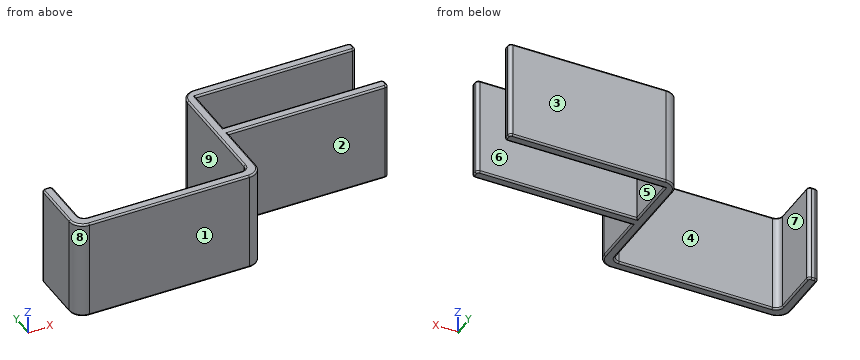
from build123d import *

# Parameters (mm, degrees)
PAD_DEPTH = 30
FILLET_R  = 0.5


with BuildPart() as part:
    # Sketch → Pad (new body)
    with BuildSketch(Plane(origin=(0, 0, 0), x_dir=(-1, 0, 0), z_dir=(0, 0, 1))):
        with BuildLine():
            ThreePointArc((1, 23), (-1.828427, 21.828427), (-3, 19))
            Line((-3, 3), (-3, 19))
            Line((-3, 3), (-49.999999, 3))
            ThreePointArc((-49.999999, 3), (-50.707106, 2.707107), (-50.999999, 2))
            Line((-50.999999, 1), (-50.999999, 2))
            ThreePointArc((-50.999999, 1), (-50.707106, 0.292893), (-49.999999, 0))
            Line((-3, 0), (-49.999999, 0))
            Line((-3, -16), (-3, 0))
            Line((-3, -16), (-49.999999, -16))
            ThreePointArc((-49.999999, -16), (-50.707106, -16.292893), (-50.999999, -17))
            Line((-50.999999, -18), (-50.999999, -17))
            ThreePointArc((-50.999999, -18), (-50.707106, -18.707107), (-49.999999, -19))
            Line((-4, -19), (-49.999999, -19))
            ThreePointArc((-4, -19), (-1.171573, -17.828427), (0, -15))
            Line((0, -15), (0, 18))
            ThreePointArc((2, 20), (0.585786, 19.414214), (0, 18))
            Line((2, 20), (48, 20))
            ThreePointArc((50, 18), (49.414214, 19.414214), (48, 20))
            Line((50, 18), (50, 4))
            ThreePointArc((50, 4), (50.292893, 3.292893), (51, 3))
            Line((52, 3), (51, 3))
            ThreePointArc((52, 3), (52.707107, 3.292893), (53, 4))
            Line((53, 19), (53, 4))
            ThreePointArc((53, 19), (51.828427, 21.828427), (49, 23))
            Line((1, 23), (49, 23))
        make_face()
    extrude(amount=PAD_DEPTH)

    # Fillet
    fillet_edges = [part.edges().sort_by_distance(p)[0] for p in [
        (-51.828427, -21.828427, 0),
        (-25, -23, 0),
        (1.828427, -21.828427, 0),
        (3, -11, 0),
        (26.5, -3, 0),
        (50.707106, -2.707107, 0),
        (50.999999, -1.5, 0),
        (50.707106, -0.292893, 0),
        (26.5, 0, 0),
        (3, 8, 0),
        (26.5, 16, 0),
        (50.707106, 16.292893, 0),
        (50.999999, 17.5, 0),
        (50.707106, 18.707107, 0),
        (27, 19, 0),
        (1.171573, 17.828427, 0),
        (0, -1.5, 0),
        (-0.585786, -19.414214, 0),
        (-25, -20, 0),
        (-49.414214, -19.414214, 0),
        (-50, -11, 0),
        (-50.292893, -3.292893, 0),
        (-51.5, -3, 0),
        (-52.707107, -3.292893, 0),
        (-53, -11.5, 0),
        (-51.828427, -21.828427, 30),
        (-25, -23, 30),
        (1.828427, -21.828427, 30),
        (3, -11, 30),
        (26.5, -3, 30),
        (50.707106, -2.707107, 30),
        (50.999999, -1.5, 30),
        (50.707106, -0.292893, 30),
        (26.5, 0, 30),
        (3, 8, 30),
        (26.5, 16, 30),
        (50.707106, 16.292893, 30),
        (50.999999, 17.5, 30),
        (50.707106, 18.707107, 30),
        (27, 19, 30),
        (1.171573, 17.828427, 30),
        (0, -1.5, 30),
        (-0.585786, -19.414214, 30),
        (-25, -20, 30),
        (-49.414214, -19.414214, 30),
        (-50, -11, 30),
        (-50.292893, -3.292893, 30),
        (-51.5, -3, 30),
        (-52.707107, -3.292893, 30),
        (-53, -11.5, 30),
    ]]
    fillet(fillet_edges, radius=FILLET_R)


solid = part.part
Check sheet for the modelled part. Datum: model origin and axes. Units: mm. Face numbers are marked on the shaded views. A direction names the side the tool comes from. Give positions to 0.01 mm unless a question says otherwise; leave off trailing zeros. Loops run counter-clockwise (first coordinate to the right, second up) from the corner with the lowest first, then second, coordinate; pieces in that order, holes last. Notation, with made-up numbers: M -8,4 L 38,4 A31 ccw 38,28 Z; hole C -2.75,40 d9. An arc over 180 degrees is marked long. Answer as a JSON object with one key per item and string values. Group by question number.
Q1. Cross-section at D-D on x = -26. Record the cut outline in (y, z).
Q2. Cross-section at A-A on y = -9.5. Record the cut outline in (x, z), then the cut area to 3 significant figures.
Q3. Cross-section at C-C on z = 22.5. Record the cut outline in (x, y), then the cut area to 3 significant figures.
Q4. Cross-section at B-B on x = 29. Record the cut outline in (y, z), then the cut area to 3 significant figures.
Q5. Release check for a two-part mould opening along X. For the marked faces 6, 7, 8 and 9 record: released by +X, released by -X, zero draft, split by the parting line, or undercut.
Q6. Access from +Z, -Z, +X, -X, +Y, -Y to the whole of each face (thin tool, end or side, straight path). Record for the marked faces 1, 2, 3, 4 and 5.
Q7. Material ranges on line 1 along Y through (x, z) = (33, 1.5); line 2 along X through (y, z) = (-10.5, 17.5); line 3 along X through (y, z) = (7.5, 20.25), recorded low to high. Write a range as [from, to].
Q8. Go/stop test with flat-tipped pins: P1, Ø14.5, axis at x = 24.5, z = 15.5, coming from the -Y side; P2, Ø6, axis at y = 12.5, z = 7.5, coming from the +X side; P3, Ø1.1, axis at x = -51.5, z = 9.5, coming from the +Y side. Record where each tip stops, or that it passes through.
Evaluation:
{
 "1": {"outline": "M -23,0.5 A0.5 ccw -22.5,0 L -20.5,0 A0.5 ccw -20,0.5 L -20,29.5 A0.5 ccw -20.5,30 L -22.5,30 A0.5 ccw -23,29.5 Z"},
 "2": {"outline": "M -53,0.5 A0.5 ccw -52.5,0 L -50.5,0 A0.5 ccw -50,0.5 L -50,29.5 A0.5 ccw -50.5,30 L -52.5,30 A0.5 ccw -53,29.5 Z; M 0,0.5 A0.5 ccw 0.5,0 L 2.5,0 A0.5 ccw 3,0.5 L 3,29.5 A0.5 ccw 2.5,30 L 0.5,30 A0.5 ccw 0,29.5 Z", "area": "180 mm2"},
 "3": {"outline": "M -53,-19 A4 ccw -49,-23 L -1,-23 A4 ccw 3,-19 L 3,-3 L 50,-3 A1 ccw 51,-2 L 51,-1 A1 ccw 50,0 L 3,0 L 3,16 L 50,16 A1 ccw 51,17 L 51,18 A1 ccw 50,19 L 4,19 A4 ccw 0,15 L 0,-18 A2 cw -2,-20 L -48,-20 A2 cw -50,-18 L -50,-4 A1 ccw -51,-3 L -52,-3 A1 ccw -53,-4 Z", "area": "614 mm2"},
 "4": {"outline": "M -3,0.5 A0.5 ccw -2.5,0 L -0.5,0 A0.5 ccw 0,0.5 L 0,29.5 A0.5 ccw -0.5,30 L -2.5,30 A0.5 ccw -3,29.5 Z; M 16,0.5 A0.5 ccw 16.5,0 L 18.5,0 A0.5 ccw 19,0.5 L 19,29.5 A0.5 ccw 18.5,30 L 16.5,30 A0.5 ccw 16,29.5 Z", "area": "180 mm2"},
 "5": {"face 6": "zero draft", "face 7": "undercut", "face 8": "released by -X", "face 9": "undercut"},
 "6": {"face 1": "+Z, -Z, +X, -X, -Y", "face 2": "+Z, -Z, +X, -Y", "face 3": "+Z, -Z, +X, -X, +Y", "face 4": "+Z, -Z, +Y", "face 5": "+Z, -Z, +X"},
 "7": {"line 1": "y = [-3, 0], [16, 19]", "line 2": "x = [-53, -50], [0, 3]", "line 3": "x = [0, 3]"},
 "8": {"P1": "stops at y = -3", "P2": "stops at x = 3", "P3": "stops at y = -3"}
}
